Could you check a few things on this drawing? It's one solid part, dimensions in mm from its lowest x, y, z. A direction names the side the tool comes from. Coordinates: 2 decimals unless noted, no trailing zeros. Loops run counter-clockwise (first coordinate to the right, second up) from the corner with the lowest first, then second, coordinate; pieces in that order, holes last. Notation, with made-up numbers: (-19.75, 6) -> (27.25, 6) arc R14 ccw to (27.25, 26) -> close; hole circle Ø10 at (39, 8). An arc over 180 degrees is marked (long way). One line per question, with ' | ' between items.
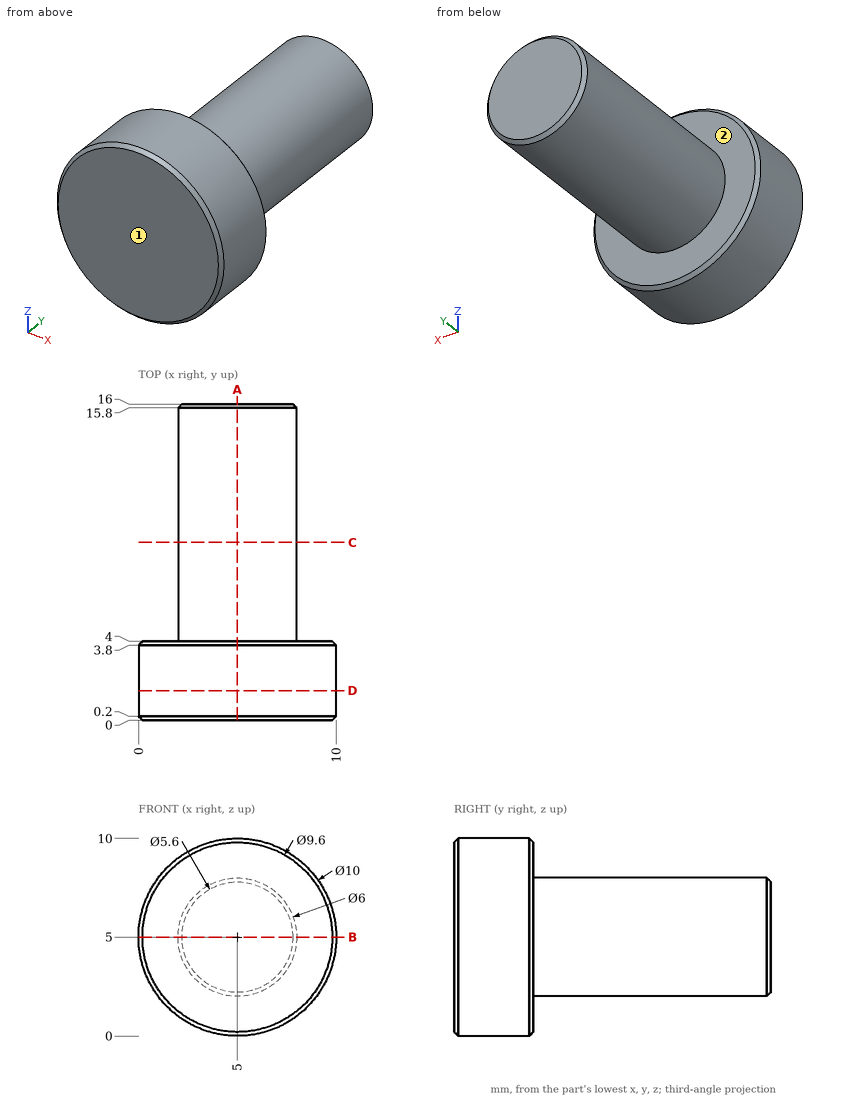
1) If we section it at A-A on x = 5: Please give me the cut outline in (y, z).
Data:
outline: (0, 0.2) -> (0.2, 0) -> (3.8, 0) -> (4, 0.2) -> (4, 2) -> (15.8, 2) -> (16, 2.2) -> (16, 7.8) -> (15.8, 8) -> (4, 8) -> (4, 9.8) -> (3.8, 10) -> (0.2, 10) -> (0, 9.8) -> close
2) If we section it at B-B on z = 5: Please give me the cut outline in (x, y), and give its area (3 significant figures).
Data:
outline: (0, 0.2) -> (0.2, 0) -> (9.8, 0) -> (10, 0.2) -> (10, 3.8) -> (9.8, 4) -> (8, 4) -> (8, 15.8) -> (7.8, 16) -> (2.2, 16) -> (2, 15.8) -> (2, 4) -> (0.2, 4) -> (0, 3.8) -> close | area: 112 mm²
3) If we section it at D-D on y = 1.5: Please give me the cut outline in (x, z).
Data:
outline: circle Ø10 at (5, 5)
4) On a 3-axis mill with a long thin cutter (end or side, diameter ignored), from which of +Z, -Z, +X, -X, +Y, -Y can I reach the whole of each face in a straight line? I mean the marked faces 1 and 2. Say none if no direction works.
Data:
face 1: +Z, -Z, +X, -X, -Y | face 2: +Y
5) If we section it at C-C on y = 9: Please give me the cut outline in (x, z), and give its area (3 significant figures).
Data:
outline: circle Ø6 at (5, 5) | area: 28.3 mm²
6) I'm going to push flat-ended pins straight in: pin 1 Ø3 at (y, z) = (3.5, 2.5) entering from -X; pin 2 Ø2 at (y, z) = (8, 2) entering from -X; pin 3 Ø2 at (x, z) = (8.5, 7.5) entering from +Y. Where does each tip first touch, or does it pass through?
Data:
pin 1: x = 0.1 | pin 2: x = 2.76 | pin 3: y = 4
7) I need wall thicknesses on line 1 along X through (y, z) = (3.75, 9); line 2 along Y through (x, z) = (3.5, 8). Which ranges of each line are inside material? Lowest first, please. Write a range as from..to.
Data:
line 1: 2..8 | line 2: 0..4
